Read the model definition and answer for the solid it produces. Units are mm, in the model's axes. Face numbers are marked on the shaded views. A direction names the side the tool comes from. Give positions to 0.01 mm unless a question says otherwise; leave off trailing zeros. Order: outer loops, then holes, each group sorted by start corner. A loop starts at its lowest first (then second) coordinate and runs counter-clockwise, first axis right, second up. Notation, with made-up numbers: (50.25, -17.75) - (105.25, -17.75) arc R38 ccw to (105.25, 20.25) - close; hole circle Ø1 at (-37, 51). An arc over 180 degrees is marked (long way). Write item = value, one per line.
```python
from build123d import *

# Parameters (mm, degrees)
SKETCH1_R           = 3
SKETCH1_R_2         = 1.5
BOSS_EXTRUDE1_DEPTH = 2.5
SKETCH2_R           = 2.75
SKETCH2_R_2         = 1.75
CUT_EXTRUDE1_DEPTH  = 0.25
CUT_EXTRUDE2_START  = -2.25
SKETCH2_2_R         = 2.75
SKETCH2_2_R_2       = 1.75
CUT_EXTRUDE2_DEPTH  = 0.25
FILLET1_R           = 0.125
CHAMFER1_SIZE       = 0.25


with BuildPart() as part:
    # Sketch1 → Boss-Extrude1 (new body)
    with BuildSketch(Plane.XY):
        Circle(SKETCH1_R)
        Circle(SKETCH1_R_2, mode=Mode.SUBTRACT)
    extrude(amount=BOSS_EXTRUDE1_DEPTH)

    # Sketch2 → Cut-Extrude1 (cut)
    with BuildSketch(Plane.XY.offset(2.5)):
        Circle(SKETCH2_R)
        Circle(SKETCH2_R_2, mode=Mode.SUBTRACT)
    extrude(amount=-CUT_EXTRUDE1_DEPTH, mode=Mode.SUBTRACT)

    # Sketch2<2> → Cut-Extrude2 (cut)
    with BuildSketch(Plane.XY.offset(2.5).offset(CUT_EXTRUDE2_START)):
        Circle(SKETCH2_2_R)
        Circle(SKETCH2_2_R_2, mode=Mode.SUBTRACT)
    extrude(amount=-CUT_EXTRUDE2_DEPTH, mode=Mode.SUBTRACT)

    # Fillet1
    fillet1_edges = [part.edges().sort_by_distance(p)[0] for p in [
        (-3, 0, 0),
        (-3, 0, 2.5),
        (-1.5, 0, 0),
        (-1.5, 0, 2.5),
    ]]
    fillet(fillet1_edges, radius=FILLET1_R)

    # Chamfer1
    chamfer1_edges = [part.edges().sort_by_distance(p)[0] for p in [
        (-2.75, 0, 2.25),
        (-1.75, 0, 2.25),
        (-2.75, 0, 0.25),
        (-1.75, 0, 0.25),
    ]]
    chamfer(chamfer1_edges, length=CHAMFER1_SIZE - 0.0001)  # a hair under: the kernel refuses the full size


solid = part.part
```
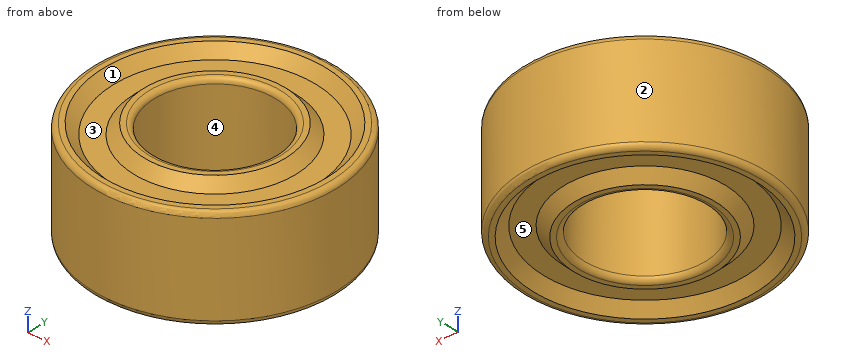
1. Straight lines are drawn through the part: L1, parallel to Y at x = 0, z = 1; L2, parallel to Y at x = -2.25, z = 0.15; L3, parallel to X at y = 1.25, z = 1.3. For each, find the intervals that lie inside material, in ascending order. Write a range as [from, to].
Recorded:
L1 = [-3, -1.5], [1.5, 3]
L2 = [-1.98, -1.3], [1.3, 1.98]
L3 = [-2.73, -0.83], [0.83, 2.73]
2. For the marked faces 3, 4 and 5, determine the directions among +Z, -Z, +X, -X, +Y, -Y from which every point of the face is accessible in a straight line to the end or side of a thin tool.
Recorded:
face_3 = +Z
face_4 = +Z, -Z
face_5 = -Z
3. Section A-A (z = 0.85) is taken. Determine the outline of the cut face in (x, y).
Recorded:
outline = circle Ø6 at (0, 0); hole circle Ø3 at (0, 0)
4. Flat-ended cylindrical pins translate along their axes: pin 1 (1 mm diameter, centred on x = 2, y = 1.5, fed in from +Z); pin 2 (1.5 mm diameter, centred on x = 0, y = -0.5, fed in from -Z); pin 3 (1 mm diameter, centred on x = 2, z = 1.5, fed in from -Y); pin 4 (1 mm diameter, centred on y = 1, z = 1.5, fed in from +X). Find the tip coordinate at first contact, or state that the pin passes through.
Recorded:
pin_1 = 2.5
pin_2 = through
pin_3 = -2.6
pin_4 = 2.96
5. Determine the mould class of the marked faces 1 and 2 for opening direction Y: +Y half, -Y half, draft (parallel to the pull), parting line (faces both ways), or undercut.
Recorded:
face_1 = undercut
face_2 = parting line
